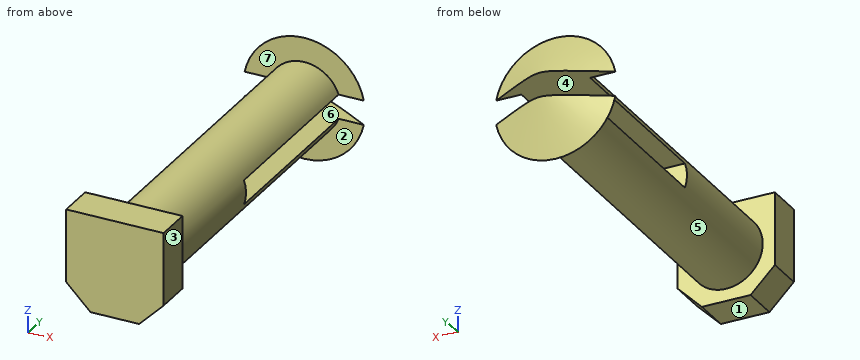
Autodesk Inventor part; units mm, degrees
ref_plane "YZ Plane" through (0, 0, 0) normal (1, 0, 0) x (0, 1, 0)
ref_plane "XZ Plane" through (0, 0, 0) normal (0, 1, 0) x (-1, 0, 0)
ref_plane "XY Plane" through (0, 0, 0) normal (0, 0, 1) x (1, 0, 0)
sketch "Boceto1" plane through (0, 0, 0) normal (1, 0, 0) x (0, 1, 0)
  line L0 (0, 0) -> (0, 3)
  line L1 (0, 3) -> (27, 3)
  line L2 (27, 0) -> (0, 0)
  line L3 (27, 0) -> (30, 0)
  line L4 (30, 0) -> (27, 5)
  line L5 (27, 5) -> (27, 3)
  dimension "d0" = 3
  dimension "d1" = 27
  dimension "d2" = 5
revolve "Revolución1" add sketch "Boceto1" angle 360 about axis through (0, 27, 0) along (0, -1, 0)
sketch "Boceto2" plane through (0, 0, 0) normal (0, -1, 0) x (1, 0, 0)
  line L0 (0, 0) -> (4, 0)
  line L1 (4, 0) -> (4, 4)
  line L2 (4, 4) -> (-4, 4)
  line L3 (-4, 4) -> (-4, -4)
  line L4 (-4, -4) -> (4, -4)
  line L5 (4, -4) -> (4, 0)
  line L6 (4, -4) -> (4, -2)
  line L7 (4, -4) -> (2, -4)
  line L8 (2, -4) -> (4, -2)
  line L9 (-4, -4) -> (-4, -2)
  line L10 (-4, -4) -> (-2, -4)
  line L11 (-2, -4) -> (-4, -2)
  dimension "d5" = 4
  dimension "d6" = 4
  dimension "d7" = 8
  dimension "d8" = 8
  dimension "d9" = 2
extrude "Extrusión1" add sketch "Boceto2" along normal blind 3 contours L5 L8 L4 L11 L3 L2 L1
sketch "Boceto4" plane through (0, 0, 0) normal (1, 0, 0) x (0, 1, 0)
  line L0 (30, 0) -> (27, 0)
  line L1 (27, 0) -> (12, 0)
  line L2 (27, -5) -> (27, 5)
  line L3 (27, 0) -> (42, 0) construction
  line L4 (12, 0) -> (12, 1)
  line L5 (12, 1) -> (27, 1)
  line L6 (27, 0) -> (27, 1)
  line L7 (12, 0) -> (12, -1)
  line L8 (12, -1) -> (27, -1)
  line L9 (27, -1) -> (27, 0)
  point P0 (0, 0)
  dimension "d15" = 15
  dimension "d16" = 180
  dimension "d17" = 1
  dimension "d18" = 1
extrude "Extrusión2" cut sketch "Boceto4" along normal mid plane 7
sketch "Boceto5" plane through (0, 27, 0) normal (0, -1, 0) x (1, 0, 0)
  line L0 (-2.8284, -1) -> (2.8284, -1)
  line L1 (-2.8284, -1) -> (2.8284, -1)
  arc A0 (2.8284, 1) -> (-2.8284, 1) centre (0, 0) ccw
  line L2 (-2.8284, 1) -> (-2.8284, 1)
  line L3 (2.8284, 1) -> (2.8284, -1)
  line L4 (-2.8284, 1) -> (-2.8284, -1)
  line L5 (-2.8284, 1) -> (2.8284, 1)
  line L6 (-2.8284, 1) -> (2.8284, 1)
extrude "Extrusión3" cut sketch "Boceto5" against normal blind 7 contours L4 L5 L3 L0
sketch "Boceto6" plane through (-2.8284, 27, 1) normal (1, 0, 0) x (0, 0, -1)
  line L0 (2, 0) -> (0, 0)
  line L1 (0, 0) -> (0, 1.2)
  line L2 (0, 0) -> (0, 1.2)
  line L3 (0, 1.2) -> (0, 3.2)
  line L4 (0, 0) -> (0, -15)
  line L5 (0, 0) -> (2, 0)
  line L6 (2, 0) -> (2, 1.2)
  line L7 (2, 0) -> (2, 3.2)
  line L8 (2, 3.2) -> (0, 3.2)
  point P0 (1, -27)
  dimension "d23" = 2
extrude "Extrusión4" cut sketch "Boceto6" along normal mid plane 20
properties part number "tornillo"
Input: part model. Units: mm. Frame: model coordinates. Face numbers are marked on the shaded views. A direction names the side the tool comes from. Round coordinates to 2 decimals unless told otherwise and drop trailing zeros. Loops run counter-clockwise (first coordinate to the right, second up) from the corner with the lowest first, then second, coordinate; pieces in that order, holes last. Notation, with made-up numbers: (37, -6) -> (81, -6) arc R10 cw to (81, 10) -> close; hole circle Ø11 at (48, 36). An arc over 180 degrees is marked (long way). One line per item, written item: value.
(1) Pin query (flat end, axial travel): pin 1 (2 mm diameter, centred on y = 5, z = 3.5, fed in from +X); pin 2 (6 mm diameter, centred on y = 23, z = -0.5, fed in from +X); pin 3 (0.9 mm diameter, centred on y = -1.5, z = 1.5, fed in from -X). Return the tip coordinate at first contact, or that it passes through.
Geometry check:
pin 1: x = 1.66
pin 2: x = 2.83
pin 3: x = -4
(2) Set-up query: the marked faces 1, 2 and 3. Return all of +Z, -Z, +X, -X, +Y, -Y with unobstructed straight access to the full face (end or side cutting, diameter ignored); none if empty.
Geometry check:
face 1: -Z, +X, -X, -Y
face 2: -Z
face 3: +Z, -Z, +X, -Y
(3) Section D-D (y = 7). Return the cut outline in (x, z), plus the area to 3 significant figures.
Geometry check:
outline: circle Ø6 at (0, 0)
area: 28.3 mm2
(4) Section A-A (z = 0). Return the cut outline in (x, y), plus the area to 3 significant figures.
Geometry check:
outline: (-4, -3) -> (4, -3) -> (4, 0) -> (3, 0) -> (3, 12) -> (-3, 12) -> (-3, 0) -> (-4, 0) -> close
area: 96.0 mm2
(5) Section C-C (y = 19). Return the cut outline in (x, z).
Geometry check:
outline: (-2.83, -1) arc R3 ccw to (2.83, -1) -> close; (-2.83, 1) -> (2.83, 1) arc R3 ccw to start
(6) Mould query, pull axis Z, two halves, no side actions, for the marked faces 4, 5, 6 and 7. Classes: pulls with the +Z half, pulls with the -Z half, needs draft (parallel to the pull), parting line crosses it, or undercut.
Geometry check:
face 4: undercut
face 5: parting line crosses it
face 6: undercut
face 7: needs draft
(7) Section B-B (x = 0). Return the cut outline in (y, z), plus the area to 3 significant figures.
Geometry check:
outline: (-3, -4) -> (0, -4) -> (0, -3) -> (27, -3) -> (27, -5) -> (29.4, -1) -> (12, -1) -> (12, 1) -> (29.4, 1) -> (27, 5) -> (27, 3) -> (0, 3) -> (0, 4) -> (-3, 4) -> close
area: 166 mm2
(8) Material intervals for line 1 (Z direction, x = 0.5, y = 21.5); line 2 (X direction, y = -1, z = -3); line 3 (Y direction, x = 0.5, z = -3.75), sorted ascending. Write a range as [from, to].
Geometry check:
line 1: [-2.96, -1], [1, 2.96]
line 2: [-3, 3]
line 3: [-3, 0], [27, 27.73]
